Input: dimensioned drawing with shaded views. Units: mm. Origin: part minimum x, y, z. A direction names the side the tool comes from. Give positions to 0.01 mm unless a question says otherwise; leave off trailing zeros. Loops run counter-clockwise (first coordinate to the right, second up) from the corner with the lowest first, then second, coordinate; pieces in that order, holes last. Notation, with made-up numbers: M 74,51.25 L 108,51.25 A15 ccw 108,73.25 Z; hole C 60.25,84.5 d10. An arc over 180 degrees is marked long. Use CSV: the item, a comma, the result in double quotes. Start each with the question number.
Q1. Section B-B, the plane z = 20. Output: boundary loops of the cut face in (x, y).
Q2. Section A-A, the plane x = 12.5. Output: boundary loops of the cut face in (y, z), plus the area to 3 significant figures.
Q3. Reachability of the marked faces 1 and 2 from +Z, -Z, +X, -X, +Y, -Y: full face, straight path, thin tool, end or side. Return the list, or none.
Q4. Section C-C, the plane z = 27. Output: boundary loops of the cut face in (x, y), plus the area to 3 significant figures.
Q5. Material intervals for line 1 along Z through (x, y) = (16.25, 9.25); line 2 along Z through (x, y) = (7, 22); line 3 along X through (y, z) = (13, 9.5), sorted ascending.
Q6. Pin query (flat end, axial travel): pin 1 (1 mm diameter, centred on y = 7, z = 23, fed in from +X); pin 2 (6 mm diameter, centred on x = 21.5, y = 15.5, fed in from -Z); pin 3 (3 mm diameter, centred on x = 21.5, y = 12.5, fed in from +Z); pin 4 (4 mm diameter, centred on x = 9.5, z = 26, fed in from +Y). Return the tip coordinate at first contact, or that it passes through.
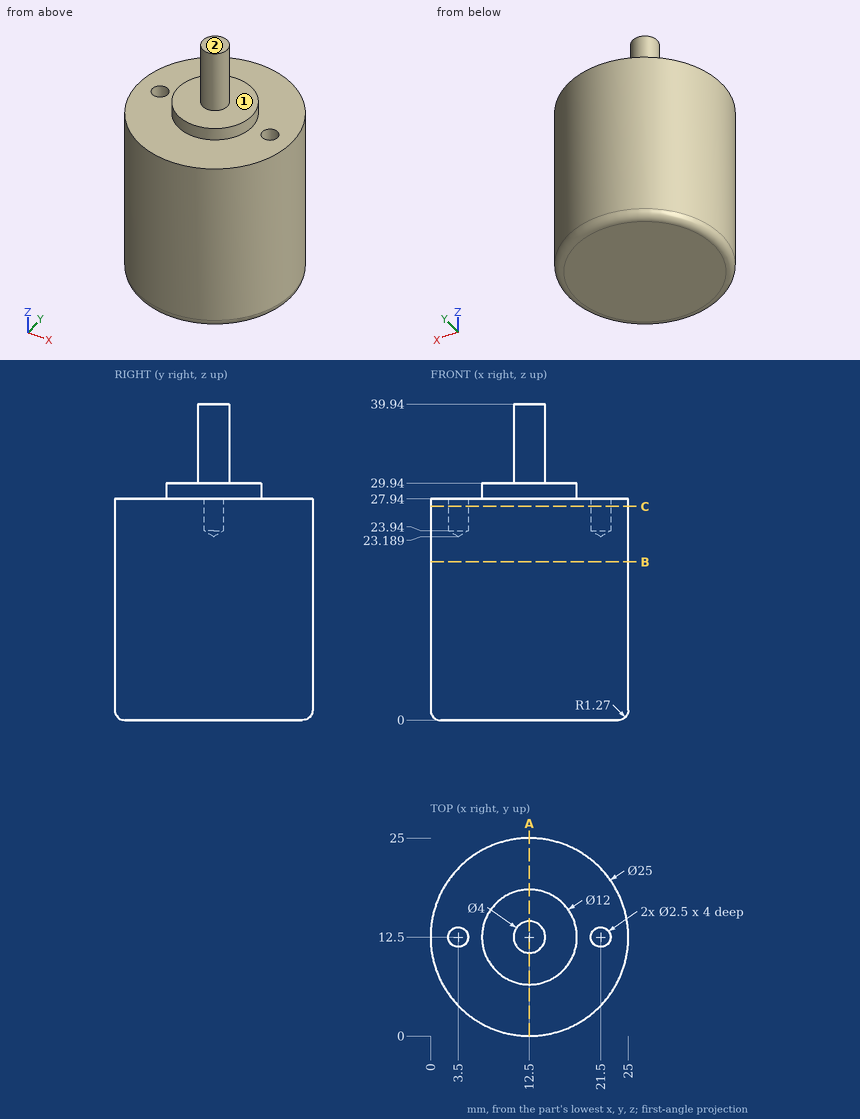
A:
1,outline,"C 12.5,12.5 d25"
2,outline,"M 0,1.27 A1.27 ccw 1.27,0 L 23.73,0 A1.27 ccw 25,1.27 L 25,27.94 L 18.5,27.94 L 18.5,29.94 L 14.5,29.94 L 14.5,39.94 L 10.5,39.94 L 10.5,29.94 L 6.5,29.94 L 6.5,27.94 L 0,27.94 Z"
2,area,"762 mm^2"
3,face 1,"+Z"
3,face 2,"+Z, +X, -X, +Y, -Y"
4,outline,"C 12.5,12.5 d25; hole C 3.5,12.5 d2.5; hole C 21.5,12.5 d2.5"
4,area,"481 mm^2"
5,line 1,"0 to 29.94"
5,line 2,"0 to 27.94"
5,line 3,"0.01 to 24.99"
6,pin 1,"x = 23.96"
6,pin 2,"z = 0"
6,pin 3,"z = 27.94"
6,pin 4,"y = 24.96"
